```python
from build123d import *

# Parameters (mm, degrees)
SKETCH1_R                = 5
BOSS_EXTRUDE1_DEPTH      = 170
BOSS_EXTRUDE2_DEPTH      = 20
BOSS_EXTRUDE2_DEPTH_BACK = 20
SKETCH2_W                = 40
SKETCH2_H                = 30
SKETCH3_W                = 35.762712216
SKETCH3_H                = 36.50555787
CUT_EXTRUDE5_DEPTH       = 16
SKETCH5_R                = 5
BOSS_EXTRUDE3_DEPTH      = 16
SKETCH8_W                = 35.762712216
SKETCH8_H                = 36.50555787
CUT_EXTRUDE7_DEPTH       = 18
SKETCH10_R               = 5
BOSS_EXTRUDE4_DEPTH      = 18
SKETCH11_W               = 80
SKETCH11_H               = 50
BOSS_EXTRUDE5_DEPTH      = 5
BOSS_EXTRUDE6_REACH      = 192.919
SKETCH13_W               = 6.494593436
SKETCH13_H               = 55.023638824
SKETCH16_W               = 8.344392414
SKETCH16_H               = 50
CUT_EXTRUDE9_DEPTH       = 10
SKETCH17_W               = 3.25
SKETCH17_H               = 8.3
CUT_EXTRUDE10_DEPTH      = 10


with BuildPart() as part:
    # Sketch1 → Boss-Extrude1 (new body)
    with BuildSketch(Plane.XY):
        Circle(SKETCH1_R)
    extrude(amount=-BOSS_EXTRUDE1_DEPTH)

    # Sketch2 → Boss-Extrude2 (add, two sides: drawn at the far end of the back side and taken through both)
    with BuildSketch(Plane(origin=(0, 0, 0), x_dir=(1, 0, 0), z_dir=(0, 1, 0)).offset(-BOSS_EXTRUDE2_DEPTH_BACK)):
        with Locations((0, 76.591812116)):
            Rectangle(SKETCH2_W, SKETCH2_H)
        with Locations((0, 129.121611958)):
            Rectangle(SKETCH2_W, SKETCH2_H)
    extrude(amount=BOSS_EXTRUDE2_DEPTH + BOSS_EXTRUDE2_DEPTH_BACK)

    # Sketch3 → Cut-Extrude5 (cut)
    with BuildSketch(Plane(origin=(0, 0, -144.121611958), x_dir=(-1, 0, 0), z_dir=(0, 0, -1))):
        Rectangle(SKETCH3_W, SKETCH3_H)
    extrude(amount=-CUT_EXTRUDE5_DEPTH, mode=Mode.SUBTRACT)


with BuildPart() as cut_extrude5_piece_1:
    # of the separate pieces the step leaves, piece 1, a body of its own (cut_extrude5_pieces)
    add(part.part.solids().sort_by_distance((5, 0, 0))[0])



with BuildPart() as cut_extrude5_piece_2:
    # of the separate pieces the step leaves, piece 2, a body of its own (cut_extrude5_pieces)
    add(part.part.solids().sort_by_distance((5, 0, -144.121611958))[0])


with BuildPart() as cut_extrude5_piece_1_1:
    add(cut_extrude5_piece_1.part)

    add(cut_extrude5_piece_2.part)  # Boss-Extrude3 merges Cut-Extrude5 piece 2
    # Sketch5 → Boss-Extrude3 (add)
    with BuildSketch(Plane(origin=(0, 0, -128.121611958), x_dir=(-1, 0, 0), z_dir=(0, 0, -1))):
        with Locations(Location((0, 0, 0), (0, 0, 180))):
            Circle(SKETCH5_R)
    extrude(amount=BOSS_EXTRUDE3_DEPTH)

    # Sketch8 → Cut-Extrude7 (cut)
    with BuildSketch(Plane(origin=(0, 0, -91.591812116), x_dir=(-1, 0, 0), z_dir=(0, 0, -1))):
        Rectangle(SKETCH8_W, SKETCH8_H)
    extrude(amount=-CUT_EXTRUDE7_DEPTH, mode=Mode.SUBTRACT)


with BuildPart() as cut_extrude7_piece_1:
    # of the separate pieces the step leaves, piece 1, a body of its own (cut_extrude7_pieces)
    add(cut_extrude5_piece_1_1.part.solids().sort_by_distance((5, 0, -144.121611958))[0])



with BuildPart() as cut_extrude7_piece_2:
    # of the separate pieces the step leaves, piece 2, a body of its own (cut_extrude7_pieces)
    add(cut_extrude5_piece_1_1.part.solids().sort_by_distance((-20, 20, -91.591812116))[0])


with BuildPart() as cut_extrude7_piece_1_1:
    add(cut_extrude7_piece_1.part)

    add(cut_extrude7_piece_2.part)  # Boss-Extrude4 merges Cut-Extrude7 piece 2
    # Sketch10 → Boss-Extrude4 (add)
    with BuildSketch(Plane(origin=(0, 0, -73.591812116), x_dir=(-1, 0, 0), z_dir=(0, 0, -1))):
        with Locations(Location((0, 0, 0), (0, 0, 180))):
            Circle(SKETCH10_R)
    extrude(amount=BOSS_EXTRUDE4_DEPTH)

    # Sketch11 → Boss-Extrude5 (add)
    with BuildSketch(Plane(origin=(0, 0, -170), x_dir=(-1, 0, 0), z_dir=(0, 0, -1))):
        Rectangle(SKETCH11_W, SKETCH11_H)
    extrude(amount=BOSS_EXTRUDE5_DEPTH)

    # Boss-Extrude6: up to this face of the body (flat: up to its plane)
    boss_extrude6_end = Plane(cut_extrude7_piece_1_1.part.faces().sort_by_distance((0, -24.056601887, -170))[0])
    # Sketch13 → Boss-Extrude6 (add, up to the picked face)
    with BuildSketch(Plane(origin=(0, 0, -185), x_dir=(-1, 0, 0), z_dir=(0, 0, -1)), mode=Mode.PRIVATE) as boss_extrude6_sk1:
        Rectangle(SKETCH13_W, SKETCH13_H)
    boss_extrude6_tool1 = split(extrude(boss_extrude6_sk1.sketch, amount=-BOSS_EXTRUDE6_REACH, mode=Mode.PRIVATE), bisect_by=boss_extrude6_end, keep=Keep.BOTH, mode=Mode.PRIVATE)
    add(boss_extrude6_tool1.solids().sort_by(Axis((0, 0, -185), (0, 0, 1)))[0])

    # Sketch16 → Cut-Extrude9 (cut)
    with BuildSketch(Plane(origin=(3.247296718, 0, 0), x_dir=(0, 0, -1), z_dir=(1, 0, 0))):
        with Locations((179.172196207, 0)):
            Rectangle(SKETCH16_W, SKETCH16_H)
    extrude(amount=-CUT_EXTRUDE9_DEPTH, mode=Mode.SUBTRACT)

    # Sketch17 → Cut-Extrude10 (cut)
    with BuildSketch(Plane(origin=(0, 0, -185), x_dir=(-1, 0, 0), z_dir=(0, 0, -1))):
        Rectangle(SKETCH17_W, SKETCH17_H)
    extrude(amount=-CUT_EXTRUDE10_DEPTH, mode=Mode.SUBTRACT)


solid = cut_extrude7_piece_1_1.part
```
Geometry check sheet. Reference: the model listing, model coordinates, mm. A direction names the side the tool comes from. Give positions to 0.01 mm unless a question says otherwise; leave off trailing zeros. Loops run counter-clockwise (first coordinate to the right, second up) from the corner with the lowest first, then second, coordinate; pieces in that order, holes last. Notation, with made-up numbers: (11.5, 22.25) - (55.5, 22.25) arc R15 cw to (55.5, 26.25) - close; hole circle Ø3 at (-4, 12.5). An arc over 180 degrees is marked (long way). Use CSV: the item, a comma, the result in double quotes. Start each with the question number.
Q1. Scan lines: probe 1 along Z at (x, y) = (18, 13.5); probe 2 along Z at (x, y) = (-6.5, 3.5); probe 3 along X at (y, z) = (0, -144). Record each from-to range of solid material in increasing order. Write a range as from..to.
Q2. Go/stop test with flat-tipped pins: pin 1 Ø5 at (x, y) = (10.5, -8) entering from -Z; pin 2 Ø12 at (x, z) = (12.5, -78.5) entering from -Y; pin 3 Ø10 at (y, z) = (-5.5, -150) entering from -X; pin 4 Ø12 at (y, z) = (-8, -177.5) entering from +X. Record where each tip stops, or that it passes through.
Q3. Access from +Z, -Z, +X, -X, +Y, -Y to the whole of each face (thin tool, end or side, straight path). Record for faces 4 (the face through (20, 0, -76)), 5 (the face through (-20, 0, -129)), 6 (the face through (-21, -25, -172)).
Q4. Section check C-C, the plane z = -65.5. Record the cut outline in (x, y).
Q5. Section check D-D, the plane y = 0. Count the separate pieces of the cut face and the enclosed holes in it, and give its area (3 significant figures).
Q6. Section check B-B, the plane y = 22.5. Record the cut outline in (x, z), and give its area (3 significant figures).
Q7. Section check A-A, the plane x = -14. Record the cut outline in (y, z), and give its area (3 significant figures).
Q8. Release check for a two-part mould opening along X. For faces 1 (the face through (-40, 0, -172)), 2 (the face through (0, -18.253, -83)), 3 (the face through (-1.08, -4.88, -30.36)) record: +X half, -X half, draft (parallel to the pull), parting line (faces both ways), or undercut.
Findings below:
1,probe 1,"z = -175..-170, -144.12..-114.12, -91.59..-61.59"
1,probe 2,"z = -175..-170, -128.12..-114.12, -73.59..-61.59"
1,probe 3,"x = -20..-17.88, -5..5, 17.88..20"
2,pin 1,"stops at z = -175"
2,pin 2,"stops at y = -20"
2,pin 3,"stops at x = -4.97"
2,pin 4,"stops at x = 40"
3,face 4,"+Z, +X, +Y, -Y"
3,face 5,"+Z, -X, +Y, -Y"
3,face 6,"+Z, -Z, -X, -Y"
4,outline,"(-20, -20) - (20, -20) - (20, 20) - (-20, 20) - close"
5,separate pieces,"3"
5,enclosed holes,"0"
5,area,"3,030 mm^2"
6,outline,"(-40, -175) - (40, -175) - (40, -170) - (-40, -170) - close; (-3.25, -185) - (3.25, -185) - (3.25, -183.34) - (-3.25, -183.34) - close"
6,area,"411 mm^2"
7,outline,"(-25, -175) - (25, -175) - (25, -170) - (-25, -170) - close; (-20, -144.12) - (-18.25, -144.12) - (-18.25, -128.12) - (18.25, -128.12) - (18.25, -144.12) - (20, -144.12) - (20, -114.12) - (-20, -114.12) - close; (-20, -91.59) - (-18.25, -91.59) - (-18.25, -73.59) - (18.25, -73.59) - (18.25, -91.59) - (20, -91.59) - (20, -61.59) - (-20, -61.59) - close"
7,area,"1,410 mm^2"
8,face 1,"-X half"
8,face 2,"undercut"
8,face 3,"parting line"
